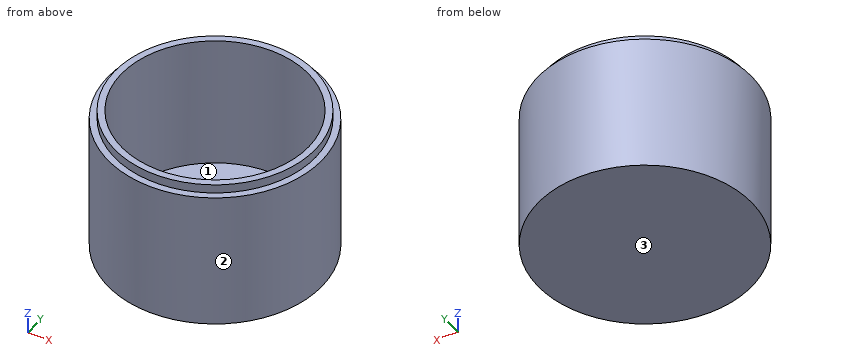
from build123d import *

# Parameters (mm, degrees)
F0_R     = 60
F1_DEPTH = 7.5
F2_R     = 60
F2_R_2   = 52.5
F3_DEPTH = 75
F4_R     = 60
F4_R_2   = 56.25
F5_DEPTH = 5


with BuildPart() as f1:
    # F0 (on Top) → F1 (new body)
    with BuildSketch(Plane.XY):
        Circle(F0_R)
    extrude(amount=F1_DEPTH)

    # F2 (on face) → F3 (join)
    with BuildSketch(Plane.XY.offset(7.5)):
        Circle(F2_R)
        Circle(F2_R_2, mode=Mode.SUBTRACT)
    extrude(amount=F3_DEPTH)

    # F4 (on face) → F5 (cut)
    with BuildSketch(Plane.XY.offset(82.5)):
        Circle(F4_R)
        Circle(F4_R_2, mode=Mode.SUBTRACT)
    extrude(amount=-F5_DEPTH, mode=Mode.SUBTRACT)


solid = f1.part
CAD build for the part. Positions are in the model's coordinates, mm. Face numbers are marked on the shaded views. Round coordinates to 2 decimals unless told otherwise and drop trailing zeros. Order: outer loops, then holes, each group sorted by start corner. A loop starts at its lowest first (then second) coordinate and runs counter-clockwise, first axis right, second up. Notation, with made-up numbers: M 28.25,48 L 80.25,48 A17 cw 80.25,72 Z; hole C 7.5,61.25 d2. An arc over 180 degrees is marked long. Use one line per item in the form item = value.
Q1. Flat gauge pins, fed straight in: P1, Ø12, axis at x = 25, z = 42.5, coming from the +Y side; P2, Ø8, axis at y = 24, z = 44.5, coming from the -X side; P3, Ø10, axis at x = -44, z = 54.5, coming from the +Y side; P4, Ø4, axis at x = 43.5, y = 8, coming from the -Z side. Where does each tip first touch, or does it go through?
Recorded:
P1 = 56.91
P2 = -56.57
P3 = 45.6
P4 = 0
Q2. Saw through at B-B on x = 0. Give the cut face in (y, z).
Recorded:
outline = M -60,0 L 60,0 L 60,77.5 L 56.25,77.5 L 56.25,82.5 L 52.5,82.5 L 52.5,7.5 L -52.5,7.5 L -52.5,82.5 L -56.25,82.5 L -56.25,77.5 L -60,77.5 Z
Q3. Two-plate mould, pull along X, no slides. Class the marked faces 1, 2 and 3: +X half, -X half, draft (parallel to the pull), parting line (faces both ways), or undercut.
Recorded:
face_1 = undercut
face_2 = parting line
face_3 = draft
Q4. Probe L1, parallel to Y at x = 0, z = 46; L2, parallel to Z at x = 25, y = -8.5; L3, parallel to Z at x = -32, y = 50. List the from-to ranges inside material, lowest first.
Recorded:
L1 = -60 to -52.5, 52.5 to 60
L2 = 0 to 7.5
L3 = 0 to 77.5
Q5. Saw through at A-A on z = 58. Give the cut face in (x, y).
Recorded:
outline = C 0,0 d120; hole C 0,0 d105
